```python
from build123d import *

# Parameters (mm, degrees)
SKETCH_1_R               = 3.5
EXTRUDE_1_DEPTH          = 90
SKETCH_2_R               = 7
EXTRUDE_2_DEPTH          = 3
FILLET_1_R               = 0.5
CUT_EXTRUDE_1_DEPTH      = 91.542807555
CUT_EXTRUDE_1_DEPTH_BACK = 91.542807555
SKETCH_3_W               = 8
SKETCH_3_H               = 1.5
SKETCH_4_W               = 39.6
SKETCH_4_H               = 1
FILLET_2_R               = 0.5
CUT_EXTRUDE_START        = -22
SKETCH_5_R               = 2.5
SKETCH_5_R_2             = 1.5
CUT_EXTRUDE_2_DEPTH      = 22
CUT_EXTRUDE_3_DEPTH      = 91.542807555
CUT_EXTRUDE_3_DEPTH_BACK = 91.542807555
SKETCH_6_R               = 1.25
SKETCH_7_R               = 4.059056145
CUT_EXTRUDE_4_DEPTH      = 12
CHAMFER_1_SIZE           = 0.3


with BuildPart() as part:
    # 草图1 → 凸台-拉伸1 (new body)
    with BuildSketch(Plane(origin=(0, 0, 0), x_dir=(0, 0, -1), z_dir=(1, 0, 0))):
        with Locations(Location((0, 0, 0), (0, 0, 180))):
            Circle(SKETCH_1_R)
    extrude(amount=EXTRUDE_1_DEPTH)

    # 草图2 → 凸台-拉伸2 (add)
    with BuildSketch(Plane.ZY):
        Circle(SKETCH_2_R)
    extrude(amount=EXTRUDE_2_DEPTH)

    # 圆角1
    fillet_1_edges = [part.edges().sort_by_distance(p)[0] for p in [
        (-3, 0, -7),
    ]]
    fillet(fillet_1_edges, radius=FILLET_1_R)

    # 草图3 → 切除-拉伸1 (cut, two sides: drawn at the far end of the back side and taken through both)
    with BuildSketch(Plane.XY.offset(-CUT_EXTRUDE_1_DEPTH_BACK)):
        with Locations((38.4, 2.75)):
            Rectangle(SKETCH_3_W, SKETCH_3_H)
    extrude(amount=CUT_EXTRUDE_1_DEPTH + CUT_EXTRUDE_1_DEPTH_BACK, mode=Mode.SUBTRACT)

    # 草图4 → 切除-旋转1 (revolve, cut)
    with BuildSketch(Plane.XY, mode=Mode.PRIVATE) as cut_revolve_1_sk:
        with Locations((70.2, 3)):
            Rectangle(SKETCH_4_W, SKETCH_4_H)
    revolve(cut_revolve_1_sk.sketch.rotate(Axis((34.4, 0, 0), (1, 0, 0)), 90), axis=Axis((34.4, 0, 0), (1, 0, 0)), mode=Mode.SUBTRACT)

    # 圆角2
    fillet_2_edges = [part.edges().sort_by_distance(p)[0] for p in [
        (50.4, 0, -3.5),
    ]]
    fillet(fillet_2_edges, radius=FILLET_2_R)

    # 草图5 → 切除-拉伸2 (cut)
    with BuildSketch(Plane(origin=(90, 0, 0), x_dir=(0, 0, -1), z_dir=(1, 0, 0)).offset(CUT_EXTRUDE_START)):
        with Locations(Location((0, 0, 0), (0, 0, 180))):
            Circle(SKETCH_5_R)
        Circle(SKETCH_5_R_2, mode=Mode.SUBTRACT)
    extrude(amount=CUT_EXTRUDE_2_DEPTH, mode=Mode.SUBTRACT)

    # 草图6 → 切除-拉伸3 (cut, two sides: drawn at the far end of the back side and taken through both)
    with BuildSketch(Plane.XY.offset(-CUT_EXTRUDE_3_DEPTH_BACK)):
        with Locations((65, 0)):
            Circle(SKETCH_6_R)
    extrude(amount=CUT_EXTRUDE_3_DEPTH + CUT_EXTRUDE_3_DEPTH_BACK, mode=Mode.SUBTRACT)

    # 草图7 → 切除-拉伸4 (cut)
    with BuildSketch(Plane(origin=(90, 0, 0), x_dir=(0, 0, -1), z_dir=(1, 0, 0))):
        Circle(SKETCH_7_R)
    extrude(amount=-CUT_EXTRUDE_4_DEPTH, mode=Mode.SUBTRACT)

    # 倒角1
    chamfer_1_edges = [part.edges().sort_by_distance(p)[0] for p in [
        (78, 0, 1.5),
    ]]
    chamfer(chamfer_1_edges, length=CHAMFER_1_SIZE)


solid = part.part
```
CAD build for the part. Positions are in the model's coordinates, mm. A direction names the side the tool comes from. Round coordinates to 2 decimals unless told otherwise and drop trailing zeros. Loops run counter-clockwise (first coordinate to the right, second up) from the corner with the lowest first, then second, coordinate; pieces in that order, holes last. Notation, with made-up numbers: M 25,-4 L 38,-4 A12 cw 38,14 Z; hole C 33,-22.5 d6. An arc over 180 degrees is marked long. Return JSON: item names as keys, results as strings. Group by question number.
(1) Mould opens along X. For faces 1 (the cylindrical face through (-1.232, -2.681, 6.466)), 2 (the cylindrical face through (65.672, 1.054, -0.037)), 3 (the flat face through (68, 2, 0)) say: +X half, -X half, draft (parallel to the pull), parting line (faces both ways), or undercut.
(2) Saw through at D-D, the plane x = 5. List the corners of the cut face in (y, z), and give its area (3 significant figures).
(3) Tool access for faces 4 (the flat face through (50.4, -2, 2)), 5 (the flat face through (42.4, 3, 0)), 6 (the flat face through (78, 0, 0)): list every direction of +Z, -Z, +X, -X, +Y, -Y with a clear straight run to the whole face (end or side of a thin tool).
(4) Saw through at A-A, the plane y = 0. List the corners of the cut face in (x, z), and give its area (3 significant figures).
(5) Wall check: probe 1 along X at (y, z) = (0, -0.7); probe 2 along X at (y, z) = (-6, 2); probe 3 along Y at (x, z) = (38, 2). Give the ranges that are in metal, low to high. Write a range as [from, to].
(6) Saw through at C-C, the plane x = 65. List the corners of the cut face in (y, z), and give its area (3 significant figures).
(7) Drop flat-ended pins along their axis: P1, Ø0.8, axis at y = 3, z = -0.5, coming from the +X side; P2, Ø3, axis at x = 37, z = 1, coming from the +Y side; P3, Ø6, axis at x = 36.5, z = 0, coming from the +Y side; P4, Ø1.5, axis at x = 65, y = 0, coming from the -Z side. Give the stop position or say it passes through.
(8) Saw through at B-B, the plane z = 0. List the corners of the cut face in (x, y), and give its area (3 significant figures).
Answer list:
{
 "1": {"face 1": "draft", "face 2": "undercut", "face 3": "+X half"},
 "2": {"outline": "C 0,0 d7", "area": "38.5 mm2"},
 "3": {"face 4": "+X", "face 5": "+Z, -Z, +Y", "face 6": "+Z, -Z, +X, +Y, -Y"},
 "4": {"outline": "M -3,-6.5 A0.5 ccw -2.5,-7 L 0,-7 L 0,-3.5 L 49.9,-3.5 A0.5 ccw 50.4,-3 L 50.4,-2.5 L 63.75,-2.5 L 63.75,2.5 L 50.4,2.5 L 50.4,3 A0.5 ccw 49.9,3.5 L 0,3.5 L 0,7 L -2.5,7 A0.5 ccw -3,6.5 Z; M 66.25,-2.5 L 68,-2.5 L 68,-1.5 L 77.7,-1.5 L 78,-1.2 L 78,1.2 L 77.7,1.5 L 68,1.5 L 68,2.5 L 66.25,2.5 Z", "area": "500 mm2"},
 "5": {"probe 1": "[-3, 63.75], [66.25, 78]", "probe 2": "[-3, 0]", "probe 3": "[-2.87, 2]"},
 "6": {"outline": "M -1.25,-2.17 L -1.25,2.17 A2.5 ccw Z; M 1.25,-2.17 A2.5 ccw 1.25,2.17 Z", "area": "7.68 mm2"},
 "7": {"P1": "x = 50.4", "P2": "y = 2", "P3": "y = 3.5", "P4": "through"},
 "8": {"outline": "M -3,-6.5 A0.5 ccw -2.5,-7 L 0,-7 L 0,-3.5 L 49.9,-3.5 A0.5 ccw 50.4,-3 L 50.4,-2.5 L 68,-2.5 L 68,-1.5 L 77.7,-1.5 L 78,-1.2 L 78,1.2 L 77.7,1.5 L 68,1.5 L 68,2.5 L 50.4,2.5 L 50.4,3 A0.5 ccw 49.9,3.5 L 42.4,3.5 L 42.4,2 L 34.4,2 L 34.4,3.5 L 0,3.5 L 0,7 L -2.5,7 A0.5 ccw -3,6.5 Z; hole C 65,0 d2.5", "area": "496 mm2"}
}
